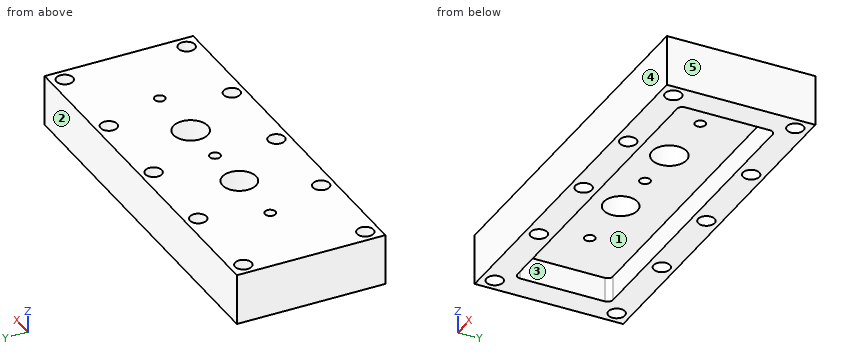
```python
from build123d import *

# Parameters (mm, degrees)
F0_W     = 71
F0_H     = 28
F0_R     = 1.55
F0_W_2   = 61
F0_H_2   = 18
F0_R_2   = 1
F0_R_3   = 3.175
F0_R_4   = 3.25
F1_DEPTH = 9.65
F2_DEPTH = 4.65
F3_R     = 1


with BuildPart() as f1:
    # F0 (on Top) → F1 (new body)
    with BuildSketch(Plane.XY):
        Rectangle(F0_W, F0_H)
        with Locations((-33, -11.5)):
            Circle(F0_R, mode=Mode.SUBTRACT)
        with Locations((-16.5, -11.593945)):
            Circle(F0_R, mode=Mode.SUBTRACT)
        with Locations((0, -11.580119)):
            Circle(F0_R, mode=Mode.SUBTRACT)
        with Locations((16.5, -11.593945)):
            Circle(F0_R, mode=Mode.SUBTRACT)
        with Locations((33, -11.5)):
            Circle(F0_R, mode=Mode.SUBTRACT)
        with Locations((-33, 11.5)):
            Circle(F0_R, mode=Mode.SUBTRACT)
        with Locations((-16.5, 11.593945)):
            Circle(F0_R, mode=Mode.SUBTRACT)
        Rectangle(F0_W_2, F0_H_2, mode=Mode.SUBTRACT)
        with Locations((0, 11.580119)):
            Circle(F0_R, mode=Mode.SUBTRACT)
        with Locations((16.5, 11.593945)):
            Circle(F0_R, mode=Mode.SUBTRACT)
        with Locations((33, 11.5)):
            Circle(F0_R, mode=Mode.SUBTRACT)
        Rectangle(F0_W_2, F0_H_2)
        with Locations((-20.4, 0)):
            Circle(F0_R_2, mode=Mode.SUBTRACT)
        with Locations((-9, 0)):
            Circle(F0_R_3, mode=Mode.SUBTRACT)
        Circle(F0_R_2, mode=Mode.SUBTRACT)
        with Locations((9, 0)):
            Circle(F0_R_4, mode=Mode.SUBTRACT)
        with Locations((20.4, 0)):
            Circle(F0_R_2, mode=Mode.SUBTRACT)
    extrude(amount=F1_DEPTH)

    # F0 (on Top) → F2 (cut)
    with BuildSketch(Plane.XY):
        Rectangle(F0_W_2, F0_H_2)
        with Locations((-20.4, 0)):
            Circle(F0_R_2, mode=Mode.SUBTRACT)
        with Locations((-9, 0)):
            Circle(F0_R_3, mode=Mode.SUBTRACT)
        Circle(F0_R_2, mode=Mode.SUBTRACT)
        with Locations((9, 0)):
            Circle(F0_R_4, mode=Mode.SUBTRACT)
        with Locations((20.4, 0)):
            Circle(F0_R_2, mode=Mode.SUBTRACT)
    extrude(amount=F2_DEPTH, mode=Mode.SUBTRACT)

    # F3
    f3_edges = [f1.edges().sort_by_distance(p)[0] for p in [
        (-30.5, -9, 2.325),
        (30.5, -9, 2.325),
        (-30.5, 9, 2.325),
        (30.5, 9, 2.325),
    ]]
    fillet(f3_edges, radius=F3_R)


solid = f1.part
```
Design review of the part built by this model. Coordinates are the model's own, in mm. Face numbers are marked on the shaded views. A direction names the side the tool comes from. Give positions to 0.01 mm unless a question says otherwise; leave off trailing zeros. Loops run counter-clockwise (first coordinate to the right, second up) from the corner with the lowest first, then second, coordinate; pieces in that order, holes last. Notation, with made-up numbers: (-20, 28) -> (-5, 28) arc R8 ccw to (-5, 34) -> close; hole circle Ø1 at (71.5, -26.75). An arc over 180 degrees is marked (long way). Write each question's results on one line, items separated by ' | '.
Q1. Machinability: for the marked faces 1 and 2, which of the approach directions +Z, -Z, +X, -X, +Y, -Y give a long, thin tool a straight path to every point of the face, cutting with its end or side? Answer none if there is none.
Reply:
face 1: -Z | face 2: +Z, -Z, +X, -X, +Y
Q2. Take a section at C-C, the plane y = 2.25. Write out the cut boundary in (x, z), plus the area to 3 significant figures.
Reply:
outline: (-35.5, 0) -> (-30.5, 0) -> (-30.5, 4.65) -> (-11.24, 4.65) -> (-11.24, 9.65) -> (-35.5, 9.65) -> close; (-6.76, 4.65) -> (6.65, 4.65) -> (6.65, 9.65) -> (-6.76, 9.65) -> close; (11.35, 4.65) -> (30.5, 4.65) -> (30.5, 0) -> (35.5, 0) -> (35.5, 9.65) -> (11.35, 9.65) -> close | area: 356 mm²
Q3. Take a section at B-B, the plane x = -9. Write out the cut boundary in (y, z) (3 decimals).
Reply:
outline: (-14, 0) -> (-9, 0) -> (-9, 4.65) -> (-3.175, 4.65) -> (-3.175, 9.65) -> (-14, 9.65) -> close; (3.175, 4.65) -> (9, 4.65) -> (9, 0) -> (14, 0) -> (14, 9.65) -> (3.175, 9.65) -> close
Q4. The part is to be moulded in two halves that separate along Y. For the marked faces 3, 4 and 5, say which applies: +Y half, -Y half, draft (parallel to the pull), parting line (faces both ways), or undercut.
Reply:
face 3: undercut | face 4: -Y half | face 5: draft
Q5. Take a section at D-D, the plane x = -22.5. Write out the cut boundary in (y, z), plus the area to 4 significant figures.
Reply:
outline: (-14, 0) -> (-9, 0) -> (-9, 4.65) -> (9, 4.65) -> (9, 0) -> (14, 0) -> (14, 9.65) -> (-14, 9.65) -> close | area: 186.5 mm²
Q6. Wall thickness on L1, parallel to Y at x = 16.5, z = 7.25; L2, parallel to Y at x = -8, z = 1.75; L3, parallel to X at y = -2.5, z = 2: over which ranges is each line inside the solid? List them lowest first.
Reply:
L1: y = -14 to -13.14, -10.04 to 10.04, 13.14 to 14 | L2: y = -14 to -9, 9 to 14 | L3: x = -35.5 to -30.5, 30.5 to 35.5
Q7. For pin 1 Ø8.5 at (x, y) = (-9, 0) entering from -Z, flat-tipped, find the tip position at first contact; note if it passes through.
Reply:
pin 1: stops at z = 4.65
Q8. Take a section at A-A, the plane x = 33. Write out the cut boundary in (y, z).
Reply:
outline: (-14, 0) -> (-13.05, 0) -> (-13.05, 9.65) -> (-14, 9.65) -> close; (-9.95, 0) -> (9.95, 0) -> (9.95, 9.65) -> (-9.95, 9.65) -> close; (13.05, 0) -> (14, 0) -> (14, 9.65) -> (13.05, 9.65) -> close
